```python
from build123d import *

# Parameters (mm, degrees)
SKETCH1_R                   = 61.595
SKETCH1_R_2                 = 44.45
EXTRUDE1_DEPTH              = 29.21
SKETCH2_R                   = 49
EXTRUDE2_DEPTH              = 24.13
CHAMFER2_SIZE               = 10.16
CHAMFER2_SIZE2              = 17.78
F_1_4_0_25_DIAMETER_HOLE1_D = 6.35
CIRPATTERN1_COUNT           = 4
CHAMFER1_SIZE               = 5.08
CHAMFER1_SIZE2              = 2.368842903


with BuildPart() as part:
    # Sketch1 → Extrude1 (new body)
    with BuildSketch(Plane.XY):
        Circle(SKETCH1_R)
        Circle(SKETCH1_R_2, mode=Mode.SUBTRACT)
    extrude(amount=EXTRUDE1_DEPTH)

    # Sketch2 → Extrude2 (cut)
    with BuildSketch(Plane(origin=(0, 0, 0), x_dir=(-1, 0, 0), z_dir=(0, 0, -1))):
        Circle(SKETCH2_R)
    extrude(amount=-EXTRUDE2_DEPTH, mode=Mode.SUBTRACT)

    # Chamfer2
    chamfer2_edges = [part.edges().sort_by_distance(p)[0] for p in [
        (-61.595, 0, 0),
    ]]
    chamfer2_side = [part.faces().sort_by_distance(p)[0] for p in [
        (-59.852830313, 0, 0),
    ]]
    chamfer(chamfer2_edges, length=CHAMFER2_SIZE, length2=CHAMFER2_SIZE2, reference=chamfer2_side[0])

    # 1/4 (0.25) Diameter Hole1 (through all)
    with Locations(Plane.XY.offset(29.21)):
        with Locations((0, 53.975)):
            f_1_4_0_25_diameter_hole1 = Hole(F_1_4_0_25_DIAMETER_HOLE1_D / 2)

    # CirPattern1: 1/4 (0.25) Diameter Hole1 ×4 about axis
    cirpattern1_axis = Axis((0, 0, 0), (0, 0, 1))
    for i in range(1, CIRPATTERN1_COUNT):
        add(f_1_4_0_25_diameter_hole1.rotate(cirpattern1_axis, i * 360 / CIRPATTERN1_COUNT), mode=Mode.SUBTRACT)

    # Chamfer1
    chamfer1_edges = [part.edges().sort_by_distance(p)[0] for p in [
        (-61.595, 0, 29.21),
    ]]
    chamfer1_side = [part.faces().sort_by_distance(p)[0] for p in [
        (-61.595, 0, 23.495),
    ]]
    chamfer(chamfer1_edges, length=CHAMFER1_SIZE, length2=CHAMFER1_SIZE2, reference=chamfer1_side[0])


solid = part.part
```
Read the model definition and answer for the solid it produces. Units are mm, in the model's axes. A direction names the side the tool comes from. Give positions to 0.01 mm unless a question says otherwise; leave off trailing zeros. Order: outer loops, then holes, each group sorted by start corner. A loop starts at its lowest first (then second) coordinate and runs counter-clockwise, first axis right, second up. Notation, with made-up numbers: (81, 13) -> (85, 13) arc R11 ccw to (85, 23) -> close; hole circle Ø2 at (-36.5, 77). An arc over 180 degrees is marked (long way). Write item = value, one per line.
1. Given pin 1 (12 mm diameter, centred on x = -5.5, z = 6, fed in from +Y); pin 2 (8 mm diameter, centred on y = 11, z = 20.5, fed in from +X); pin 3 (12 mm diameter, centred on y = -21, z = 7, fed in from +X), each flat-ended and moving along its own axis, determine where each tip first touches the part or whether it passes through.
Numbers:
pin_1 = 58.07
pin_2 = 61.2
pin_3 = 55.56
2. A cutting plane is placed at B-B, the plane x = 0. Write down the section's boundary in (y, z) (3 decimals).
Numbers:
outline = (-61.595, 17.78) -> (-57.15, 10.001) -> (-57.15, 29.21) -> (-59.226, 29.21) -> (-61.595, 24.13) -> close; (-50.8, 0) -> (-49, 0) -> (-49, 24.13) -> (-44.45, 24.13) -> (-44.45, 29.21) -> (-50.8, 29.21) -> close; (44.45, 24.13) -> (49, 24.13) -> (49, 0) -> (50.8, 0) -> (50.8, 29.21) -> (44.45, 29.21) -> close; (57.15, 10.001) -> (61.595, 17.78) -> (61.595, 24.13) -> (59.226, 29.21) -> (57.15, 29.21) -> close
3. For faces 4 (the face through (-50.876, 0.688, 17.646)), 5 (the face through (-26.34, 41.32, 11.9)), determine the directions among +Z, -Z, +X, -X, +Y, -Y from which every point of the face is accessible in a straight line to the end or side of a thin tool.
Numbers:
face_4 = +Z, -Z
face_5 = -Z
4. A cutting plane is placed at A-A, the plane z = 16. Write down the section's boundary in (x, y) (3 decimals).
Numbers:
outline = circle Ø121.156 at (0, 0); hole circle Ø6.35 at (-53.975, 0); hole circle Ø98 at (0, 0); hole circle Ø6.35 at (0, -53.975); hole circle Ø6.35 at (0, 53.975); hole circle Ø6.35 at (53.975, 0)
5. Straight lines are drawn through the part: line 1 along Y through (x, z) = (0, 6); line 2 along X through (y, z) = (39.5, 9.5); line 3 along X through (y, z) = (-22, 22.75). For each, find the intervals that lie inside material, in ascending order.
Numbers:
line_1 = -50.8 to -49, 49 to 50.8
line_2 = -40.9 to -29, 29 to 40.9
line_3 = -57.53 to -43.78, 43.78 to 57.53
6. The mould has two halves that part along X. Classify faces 1 (the face through (45.5, -18.8, 0)), 2 (the face through (-12.864, -57.93, 28.963)), 3 (the face through (-0.688, -50.876, 17.646)): +X half, -X half, draft (parallel to the pull), parting line (faces both ways), or undercut.
Numbers:
face_1 = draft
face_2 = parting line
face_3 = undercut
